Autodesk Inventor part; units mm, degrees
ref_plane "YZ Plane" through (0, 0, 0) normal (1, 0, 0) x (0, 1, 0)
ref_plane "XZ Plane" through (0, 0, 0) normal (0, 1, 0) x (-1, 0, 0)
ref_plane "XY Plane" through (0, 0, 0) normal (0, 0, 1) x (1, 0, 0)
sketch "Sketch1" plane through (0, 0, 0) normal (1, 0, 0) x (0, 1, 0)
  circle A0 centre (0, 0) radius 7.7343
  dimension "d0" = 15.4686
extrude "Extrusion1" add sketch "Sketch1" along normal blind 6.0198
sketch "Sketch2" plane through (6.0198, 0, 0) normal (1, 0, 0) x (0, 0, -1)
  circle A0 centre (0, 0) radius 3.9624
  dimension "d3" = 7.9248
extrude "Extrusion2" add sketch "Sketch2" along normal blind 6.985
sketch "Sketch3" plane through (0, 0, 0) normal (-1, 0, 0) x (0, 0, 1)
  arc A0 (-2.6416, -2.0232) -> (-2.6416, 2.0232) centre (0, 0) ccw
  line L0 (-2.6416, -2.0232) -> (-2.6416, 2.0232)
  dimension "d6" = 6.6548
extrude "Extrusion3" cut sketch "Sketch3" against normal through all
sketch "Sketch4" plane through (0, 0, 0) normal (-1, 0, 0) x (0, 0, 1)
  circle A0 centre (-4.2426, 4.2418) radius 1.15
  circle A1 centre (0, 0) radius 6 construction
  circle A2 centre (-4.2418, -4.2426) radius 1.15
  circle A3 centre (4.2426, -4.2418) radius 1.15
  circle A4 centre (4.2418, 4.2426) radius 1.15
  dimension "d12" = 2.3
  dimension "d21" = 12
  dimension "d24" = 360
extrude "Extrusion4" cut sketch "Sketch4" against normal through all
sketch "Sketch5" plane through (0, -2.0232, -2.6416) normal (0, 0, 1) x (1, 0, 0)
  circle A0 centre (3.0099, 2.0232) radius 1.45
  line L0 (6.0198, -5.7111) -> (6.0198, 9.7575)
  line L1 (0, 9.7575) -> (0, -5.7111)
  line L2 (6.0198, 5.9856) -> (13.0048, 5.9856) construction
  line L3 (13.0048, -1.9392) -> (13.0048, 5.9856) construction
  line L4 (6.0198, 5.9856) -> (6.0198, -1.9392) construction
  line L5 (0, 9.7575) -> (6.0198, 9.7575) construction
  line L6 (0, -5.7111) -> (6.0198, -5.7111) construction
  point P0 (0, 2.0232)
  dimension "d26" = 2.9
  dimension "d27" = 6.0198
  dimension "d28" = 3.0099
  dimension "d29" = 15.4686
  dimension "d30" = 7.7343
extrude "Extrusion5" cut sketch "Sketch5" against normal through all
equation "\"d28\" = 0.5 * d27"
equation "\"d30\" = 0.5 * d29"
properties part number "Our omiwheelinsert"
Could you check a few things on this model? Use its own coordinates, in mm. A direction names the side the tool comes from. Round coordinates to 2 decimals unless told otherwise and drop trailing zeros. Write each loop counter-clockwise with the first axis right and the second up, starting at its lowest first coordinate (ties: lowest second). Pieces come first, ordered by that corner, then holes. Notation, with made-up numbers: (2, 67) - (25, 67) arc R24 ccw to (25, 100) - close; hole circle Ø5 at (72.25, 58.25). An arc over 180 degrees is marked (long way). Use a Markdown table: item, result.
Q1. For pin 1 (5 mm diameter, centred on x = 9, y = 1, fed in from +Z); pin 2 (1.8 mm diameter, centred on y = -4.24, z = -4.24, fed in from +X); pin 3 (3 mm diameter, centred on y = 6, z = 6, fed in from +X); pin 4 (1.5 mm diameter, centred on x = 4.5, z = 1, fed in from -Y), each with a flat end and sliding along its axis, tell me the tip position at first contact or that it passes through.
Output values:
| item | result |
|---|---|
| pin 1 | z = 3.96 |
| pin 2 | through |
| pin 3 | x = 6.02 |
| pin 4 | y = -7.73 |
Q2. I want a section at A-A (y = 0). List the corners of the cut face in (x, z) for me.
Output values:
| item | result |
|---|---|
| outline | (0, -7.73) - (1.56, -7.73) - (1.56, -2.64) - (0, -2.64) - close; (0, 3.33) - (13, 3.33) - (13, 3.96) - (6.02, 3.96) - (6.02, 7.73) - (0, 7.73) - close; (4.46, -7.73) - (6.02, -7.73) - (6.02, -3.96) - (13, -3.96) - (13, -2.64) - (4.46, -2.64) - close |
Q3. I want a section at C-C (z = 4.5). List the corners of the cut face in (x, y) for me, plus the area to 3 significant figures.
Output values:
| item | result |
|---|---|
| outline | (0, -6.29) - (6.02, -6.29) - (6.02, -5.36) - (0, -5.36) - close; (0, -3.12) - (6.02, -3.12) - (6.02, 3.12) - (0, 3.12) - close; (0, 5.36) - (6.02, 5.36) - (6.02, 6.29) - (0, 6.29) - close |
| area | 48.7 mm2 |
Q4. I want a section at B-B (z = 1). List the corners of the cut face in (x, y) for me.
Output values:
| item | result |
|---|---|
| outline | (0, -7.67) - (6.02, -7.67) - (6.02, -3.83) - (13, -3.83) - (13, -3.17) - (0, -3.17) - close; (0, 3.17) - (13, 3.17) - (13, 3.83) - (6.02, 3.83) - (6.02, 7.67) - (0, 7.67) - close |
Q5. Thinking about a two-plate mould opening in Z: for faces 1 (the cylindrical face through (2.97, -1.68, 7.55)), 2 (the flat face through (13.005, 0, -3)), 3 (the flat face through (6, 0, -2.642)), which applies, released by +Z, released by -Z, zero draft, split by the parting line, or undercut?
Output values:
| item | result |
|---|---|
| face 1 | split by the parting line |
| face 2 | zero draft |
| face 3 | undercut |
Q6. Please list where these lines run through material, in increasing order: L1, parallel to Y at x = 7.25, z = 0; L2, parallel to X at y = 0, z = -5.65; L3, parallel to Y at x = 1.75, z = -4.75.
Output values:
| item | result |
|---|---|
| L1 | -3.96 to -3.33, 3.33 to 3.96 |
| L2 | 0 to 1.56, 4.46 to 6.02 |
| L3 | -6.1 to -5.27, -3.21 to -0.72, 0.72 to 3.21, 5.27 to 6.1 |
Q7. For faces 4 (the cylindrical face through (2.968, 3.222, -3.712)), 5 (the cylindrical face through (1.94, 0.98, -5.15)), 6 (the cylindrical face through (9.46, -3.93, 0.52)), which set-ups out of +Z, -Z, +X, -X, +Y, -Y let a thin tool reach every point of the face, with its end or its side?
Output values:
| item | result |
|---|---|
| face 4 | +X, -X |
| face 5 | -Z |
| face 6 | +X |
Q8. I want a section at D-D (y = 2.75). List the corners of the cut face in (x, z) for me, plus the area to 3 significant figures.
Output values:
| item | result |
|---|---|
| outline | (0, -7.23) - (6.02, -7.23) - (6.02, -2.85) - (13, -2.85) - (13, -1.87) - (0, -1.87) - close; (0, 1.87) - (13, 1.87) - (13, 2.85) - (6.02, 2.85) - (6.02, 7.23) - (0, 7.23) - close |
| area | 78.2 mm2 |
